```python
from build123d import *

# Parameters (mm, degrees)
F0_R     = 17.5393156129
F1_DEPTH = 50
F2_W     = 88.7956470251
F2_H     = 81.5360844135
F3_DEPTH = 25
F5_DEPTH = 25


with BuildPart() as f1:
    # F0 (on Top) → F1 (new body)
    with BuildSketch(Plane.XY):
        Circle(F0_R)
    extrude(amount=F1_DEPTH)

    # F2 (on Top) → F3 (join)
    with BuildSketch(Plane.XY):
        Rectangle(F2_W, F2_H)
    extrude(amount=F3_DEPTH)

    # F4 (on Right) → F5 (cut, symmetric)
    with BuildSketch(Plane.YZ):
        Polygon((-20.2884618193, 37.8846153617), (19.3269234151, 51.9230812788), (-20.2884618193, 53.4615404904), align=None)
    extrude(amount=F5_DEPTH, both=True, mode=Mode.SUBTRACT)


solid = f1.part
```
CAD build for the part. Positions are in the model's coordinates, mm. A direction names the side the tool comes from. Round coordinates to 2 decimals unless told otherwise and drop trailing zeros. Write each loop counter-clockwise with the first axis right and the second up, starting at its lowest first coordinate (ties: lowest second). Pieces come first, ordered by that corner, then holes. Notation, with made-up numbers: (-34.5, 37) - (16.5, 37) arc R24 ccw to (16.5, 72) - close; hole circle Ø4 at (85.5, 87.5). An arc over 180 degrees is marked (long way). Return JSON: item names as keys, results as strings. Group by question number.
Item 1: Band-saw the part on C-C on z = 34. List the corners of the cut face in (x, y), plus the area to 3 significant figures.
Item 2: Band-saw the part on A-A on x = 0. List the corners of the cut face in (y, z).
Item 3: Band-saw the part on B-B on y = 35. List the corners of the cut face in (x, z), plus the area to 3 significant figures.
Item 4: Flat gauge pins, fed straight in: pin 1 Ø1.5 at (x, y) = (14, -16) entering from +Z; pin 2 Ø4 at (y, z) = (-1, 33.5) entering from -X; pin 3 Ø2 at (x, y) = (-7.5, 7) entering from +Z. Where does each tip first touch, or does it go through?
Item 5: 3-axis set-ups, long thin cutter, end or side, ignore diameter. For faces 1 (the face through (-2.28, 17.39, 34.55)), 2 (the face through (-1, -40.768, 12)): which of +Z, -Z, +X, -X, +Y, -Y reach the whole face in a straight line?
Item 6: Probe probe 1 along Z at (x, y) = (1, 21); probe 2 along X at (y, z) = (0.5, 40); probe 3 along Y at (x, z) = (11, 37.5). List the from-to ranges inside material, lowest first.
Item 7: Band-saw the part on D-D on y = 0. List the corners of the cut face in (x, z).
Resolved:
{
 "1": {"outline": "circle Ø35.08 at (0, 0)", "area": "966 mm²"},
 "2": {"outline": "(-40.77, 0) - (40.77, 0) - (40.77, 25) - (17.54, 25) - (17.54, 50) - (13.9, 50) - (-17.54, 38.86) - (-17.54, 25) - (-40.77, 25) - close"},
 "3": {"outline": "(-44.4, 0) - (44.4, 0) - (44.4, 25) - (-44.4, 25) - close", "area": "2,220 mm²"},
 "4": {"pin 1": "stops at z = 25", "pin 2": "stops at x = -17.54", "pin 3": "stops at z = 47.91"},
 "5": {"face 1": "+Z", "face 2": "+Z, -Z, +X, -X, -Y"},
 "6": {"probe 1": "z = 0 to 25", "probe 2": "x = -17.53 to 17.53", "probe 3": "y = -13.66 to 13.66"},
 "7": {"outline": "(-44.4, 0) - (44.4, 0) - (44.4, 25) - (17.54, 25) - (17.54, 45.07) - (-17.54, 45.07) - (-17.54, 25) - (-44.4, 25) - close"}
}
